Check sheet for the modelled part. Datum: model origin and axes. Units: mm. A direction names the side the tool comes from. Give positions to 0.01 mm unless a question says otherwise; leave off trailing zeros. Write each loop counter-clockwise with the first axis right and the second up, starting at its lowest first coordinate (ties: lowest second). Pieces come first, ordered by that corner, then holes. Notation, with made-up numbers: M -26.5,-14 L 5.5,-14 A22 ccw 5.5,9 Z; hole C -17,-15 d5. An arc over 180 degrees is marked long. Write item = value, one per line. Start each with the question number.
1) Sectioned sample at B-B, the plane x = 177. Record the cut outline in (y, z).
2) Scan lines: L1, parallel to Y at x = 177.5, z = 75; L2, parallel to X at y = -115, z = 57; L3, parallel to Z at x = 171, y = -123. Record each from-to range of solid material in increasing order.
3) Sectioned sample at A-A, the plane z = 64.5. Record the cut outline in (x, y), then the cut area to 3 significant figures.
4) Gauge pin test, flat ends, axial feed: pin 1 (1 mm diameter, centred on x = 189.5, z = 74.5, fed in from +Y); pin 2 (2 mm diameter, centred on y = -127.5, z = 77.5, fed in from +X); pin 3 (2 mm diameter, centred on x = 180, y = -119.5, fed in from +Z). Record the tip position at first contact, or that the pin passes through.
5) Set-up check for faces 1 (the face through (166, -100.5, 66)), 2 (the face through (166, -101.5, 70)): record each of +Z, -Z, +X, -X, +Y, -Y from which the full face is reachable in a straight line by a thin tool's end or side.
6) Draft check along X on faces 3 (the face through (199, -117, 66)), 4 (the face through (166.02, -101.07, 46.6)), 5 (the face through (166.48, -104.35, 50.01)), 6 (the face through (133.504, -116.637, 65.748)). Enter one of: pulls with the +X half, pulls with the -X half, needs draft (parallel to the pull), parting line crosses it, or undercut.
from build123d import *

# Parameters (mm, degrees)
PAD002_DEPTH = 38
THICKNESS_T  = -1
FILLET002_R  = 10
FILLET003_R  = 2


with BuildPart() as part:
    # Sketch007 → Pad002 (new body)
    with BuildSketch(Plane.XY):
        with BuildLine():
            ThreePointArc((-83, 72.5), (-99.5, 56), (-83, 39.5))
            Line((-83, 39.5), (-50.5, 39.5))
            ThreePointArc((-50.5, 39.5), (-34, 56), (-50.5, 72.5))
            Line((-50.5, 72.5), (-83, 72.5))
        make_face()
    extrude(amount=PAD002_DEPTH)

    # Thickness
    thickness_openings = [part.faces().sort_by_distance(p)[0] for p in [
        (-66.75, 56, 38),
    ]]
    offset(amount=THICKNESS_T, openings=thickness_openings)

    # Fillet002
    fillet002_edges = [part.edges().sort_by_distance(p)[0] for p in [
        (-98.5, 56, 1),
        (-66.75, 40.5, 1),
        (-35, 56, 1),
        (-66.75, 71.5, 1),
    ]]
    fillet(fillet002_edges, radius=FILLET002_R)

    # Fillet003
    fillet003_edges = [part.edges().sort_by_distance(p)[0] for p in [
        (-99.5, 56, 0),
        (-66.75, 39.5, 0),
        (-34, 56, 0),
        (-66.75, 72.5, 0),
    ]]
    fillet(fillet003_edges, radius=FILLET003_R)


with BuildPart() as part_1:
    # Body002 placement: moved
    add(part.part.moved(Location((233, -173, 46))))


solid = part_1.part
Data:
q1.outline = M -133.5,48 A2 ccw -131.5,46 L -102.5,46 A2 ccw -100.5,48 L -100.5,84 L -101.5,84 L -101.5,57 A10 cw -111.5,47 L -122.5,47 A10 cw -132.5,57 L -132.5,84 L -133.5,84 Z
q2.L1 = -133.5 to -132.5, -101.5 to -100.5
q2.L2 = 133.62 to 134.63, 197.87 to 198.88
q2.L3 = 46 to 47.01
q3.outline = M 150,-133.5 L 182.5,-133.5 A16.5 ccw 182.5,-100.5 L 150,-100.5 A16.5 ccw Z; hole M 150,-132.5 L 182.5,-132.5 A15.5 ccw 182.5,-101.5 L 150,-101.5 A15.5 ccw Z
q3.area = 166 mm2
q4.pin_1 = -101.83
q4.pin_2 = 195.99
q4.pin_3 = 47
q5.face_1 = +Z, -Z, +X, -X, +Y
q5.face_2 = +Z
q6.face_3 = pulls with the +X half
q6.face_4 = needs draft
q6.face_5 = undercut
q6.face_6 = pulls with the -X half
